Read the model definition and answer for the solid it produces. Units are mm, in the model's axes. Face numbers are marked on the shaded views. Coordinates: 2 decimals unless noted, no trailing zeros. Loops run counter-clockwise (first coordinate to the right, second up) from the corner with the lowest first, then second, coordinate; pieces in that order, holes last. Notation, with made-up numbers: M 43.25,-6 L 86.25,-6 A18 cw 86.25,-2 Z; hole C 44,58 d9. An arc over 180 degrees is marked long. Use one line per item in the form item = value. Start each with the question number.
1. The part is cut by section B-B (y = 32.5). Give the vertices of the cut face in (x, z).
2. Find the intervals of material crossed by probe 1 along Y at (x, z) = (-2.05, 0); probe 2 along Y at (x, z) = (-2.25, 1.25); probe 3 along X at (y, z) = (32, -1.75), in increasing order. Write a range as [from, to].
3. The part is cut by section D-D (y = 23). Give the vertices of the cut face in (x, z), plus the area to 3 significant figures.
4. For a pull along X with two mould halves and no side action, classify the marked faces 1 and 2 as released by +X, released by -X, zero draft, split by the parting line, or undercut.
5. The part is cut by section A-A (y = -2.5). Give the number of separate pieces and of enclosed holes in the cut face, plus the area to 3 significant figures.
6. Flat-ended cylindrical pins translate along their axes: pin 1 (2.5 mm diameter, centred on y = 32.5, z = 0, fed in from -X); pin 2 (3 mm diameter, centred on y = 18.5, z = -2.5, fed in from -X); pin 3 (2.5 mm diameter, centred on x = -0.5, z = 0.5, fed in from +Y); pin 4 (0.6 mm diameter, centred on y = -3, z = -2.5, fed in from -X). Find the tip coordinate at first contact, or state that the pin passes through.
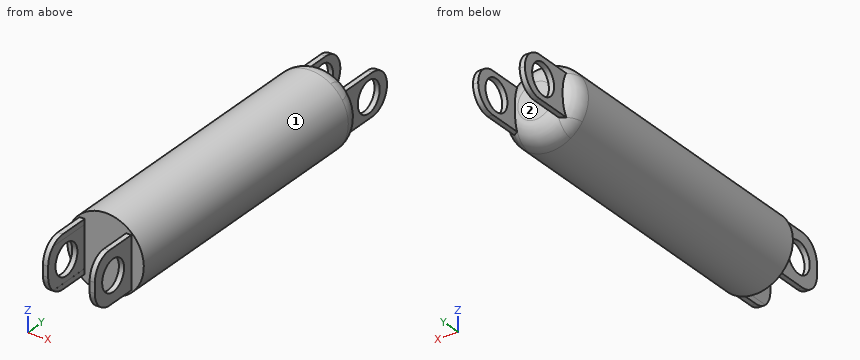
from build123d import *

# Parameters (mm, degrees)
SKETCH1_R           = 3.7
BOSS_EXTRUDE1_DEPTH = 30
SKETCH2_W           = 5
SKETCH2_H           = 4
SKETCH2_W_2         = 4
SKETCH2_H_2         = 3
BOSS_EXTRUDE2_DEPTH = 5
SKETCH3_W           = 4
SKETCH3_H           = 4.53219821
CUT_EXTRUDE1_DEPTH  = 5
SKETCH4_R           = 1.5
CUT_EXTRUDE2_DEPTH  = 15
FILLET1_R           = 2
FILLET2_R           = 2
SKETCH5_W           = 5
SKETCH5_H           = 5
SKETCH5_W_2         = 4
SKETCH5_H_2         = 4
BOSS_EXTRUDE3_DEPTH = 5
SKETCH6_W           = 3.994620944
SKETCH6_H           = 5.818695304
CUT_EXTRUDE3_DEPTH  = 5
SKETCH7_R           = 1.5
CUT_EXTRUDE4_DEPTH  = 5
FILLET3_R           = 2


# Some blends are built 0.0001 mm under size
with BuildPart() as part:
    # Sketch1 → Boss-Extrude1 (new body)
    with BuildSketch(Plane(origin=(0, 0, 0), x_dir=(1, 0, 0), z_dir=(0, 1, 0))):
        with Locations(Location((0, 0, 0), (0, 0, 270))):
            Circle(SKETCH1_R)
    extrude(amount=BOSS_EXTRUDE1_DEPTH)

    # Sketch2 → Boss-Extrude2 (add)
    with BuildSketch(Plane(origin=(0, 30, 0), x_dir=(1, 0, 0), z_dir=(0, 1, 0))):
        Rectangle(SKETCH2_W, SKETCH2_H)
        Rectangle(SKETCH2_W_2, SKETCH2_H_2, mode=Mode.SUBTRACT)
    extrude(amount=BOSS_EXTRUDE2_DEPTH)

    # Sketch3 → Cut-Extrude1 (cut)
    with BuildSketch(Plane(origin=(0, 35, 0), x_dir=(1, 0, 0), z_dir=(0, 1, 0))):
        Rectangle(SKETCH3_W, SKETCH3_H)
    extrude(amount=-CUT_EXTRUDE1_DEPTH, mode=Mode.SUBTRACT)

    # Sketch4 → Cut-Extrude2 (cut)
    with BuildSketch(Plane.ZY.offset(2.5)):
        with Locations((0, 32.5)):
            Circle(SKETCH4_R)
    extrude(amount=-CUT_EXTRUDE2_DEPTH, mode=Mode.SUBTRACT)

    # Fillet1
    fillet1_edges = [part.edges().sort_by_distance(p)[0] for p in [
        (-2.25, 35, 2),
        (-2.25, 35, -2),
        (2.25, 35, -2),
        (2.25, 35, 2),
    ]]
    fillet(fillet1_edges, radius=FILLET1_R - 0.0001)  # a hair under: the kernel refuses the full size

    # Fillet2
    # the kernel refuses this fillet: 2 mm, written as the material it takes off along each edge
    with BuildSketch(Plane(origin=(0, 30, 0), x_dir=(0, 0, 1), z_dir=(-1, 0, 0))) as fillet2_piece_1_section:
        with BuildLine():
            CenterArc((3.7 - FILLET2_R, -FILLET2_R), FILLET2_R, 0, 90)
            Line((3.7, -FILLET2_R), (3.7, 0))
            Line((3.7, 0), (3.7 - FILLET2_R, 0))
        make_face()
    fillet2_piece_1 = revolve(axis=Axis((0, 30, 0), (0, 1, 0)), mode=Mode.PRIVATE)
    fillet2_piece_1 = split(fillet2_piece_1, bisect_by=Plane(origin=(2, 29.996904363, 0.950092039), z_dir=(-1, 0, 0)), keep=Keep.TOP, mode=Mode.PRIVATE)
    fillet2_piece_1 = split(fillet2_piece_1, bisect_by=Plane(origin=(-2, 29.996904363, 0.950092039), z_dir=(1, 0, 0)), keep=Keep.TOP, mode=Mode.PRIVATE)
    add(fillet2_piece_1, mode=Mode.SUBTRACT)
    with BuildSketch(Plane(origin=(0, 30, 0), x_dir=(0, 0, 1), z_dir=(-1, 0, 0))) as fillet2_piece_2_section:
        with BuildLine():
            CenterArc((3.7 - FILLET2_R, -FILLET2_R), FILLET2_R, 0, 90)
            Line((3.7, -FILLET2_R), (3.7, 0))
            Line((3.7, 0), (3.7 - FILLET2_R, 0))
        make_face()
    fillet2_piece_2 = revolve(axis=Axis((0, 30, 0), (0, 1, 0)), mode=Mode.PRIVATE)
    fillet2_piece_2 = split(fillet2_piece_2, bisect_by=Plane(origin=(2.24397726, 29.466228533, 2), z_dir=(0, 0, 1)), keep=Keep.TOP, mode=Mode.PRIVATE)
    add(fillet2_piece_2, mode=Mode.SUBTRACT)
    with BuildSketch(Plane(origin=(0, 30, 0), x_dir=(0, 0, 1), z_dir=(-1, 0, 0))) as fillet2_piece_3_section:
        with BuildLine():
            CenterArc((3.7 - FILLET2_R, -FILLET2_R), FILLET2_R, 0, 90)
            Line((3.7, -FILLET2_R), (3.7, 0))
            Line((3.7, 0), (3.7 - FILLET2_R, 0))
        make_face()
    fillet2_piece_3 = revolve(axis=Axis((0, 30, 0), (0, 1, 0)), mode=Mode.PRIVATE)
    fillet2_piece_3 = split(fillet2_piece_3, bisect_by=Plane(origin=(2.5, 29.502863649, 1.19e-07), z_dir=(1, 0, 0)), keep=Keep.TOP, mode=Mode.PRIVATE)
    add(fillet2_piece_3, mode=Mode.SUBTRACT)
    with BuildSketch(Plane(origin=(0, 30, 0), x_dir=(0, 0, 1), z_dir=(-1, 0, 0))) as fillet2_piece_4_section:
        with BuildLine():
            CenterArc((3.7 - FILLET2_R, -FILLET2_R), FILLET2_R, 0, 90)
            Line((3.7, -FILLET2_R), (3.7, 0))
            Line((3.7, 0), (3.7 - FILLET2_R, 0))
        make_face()
    fillet2_piece_4 = revolve(axis=Axis((0, 30, 0), (0, 1, 0)), mode=Mode.PRIVATE)
    fillet2_piece_4 = split(fillet2_piece_4, bisect_by=Plane(origin=(2.243977257, 29.466228303, -2), z_dir=(0, 0, -1)), keep=Keep.TOP, mode=Mode.PRIVATE)
    add(fillet2_piece_4, mode=Mode.SUBTRACT)
    with BuildSketch(Plane(origin=(0, 30, 0), x_dir=(0, 0, 1), z_dir=(-1, 0, 0))) as fillet2_piece_5_section:
        with BuildLine():
            CenterArc((3.7 - FILLET2_R, -FILLET2_R), FILLET2_R, 0, 90)
            Line((3.7, -FILLET2_R), (3.7, 0))
            Line((3.7, 0), (3.7 - FILLET2_R, 0))
        make_face()
    fillet2_piece_5 = revolve(axis=Axis((0, 30, 0), (0, 1, 0)), mode=Mode.PRIVATE)
    fillet2_piece_5 = split(fillet2_piece_5, bisect_by=Plane(origin=(-2.5, 29.50286365, -1.18e-07), z_dir=(-1, 0, 0)), keep=Keep.TOP, mode=Mode.PRIVATE)
    add(fillet2_piece_5, mode=Mode.SUBTRACT)

    # Sketch5 → Boss-Extrude3 (add)
    with BuildSketch(Plane.XZ):
        Rectangle(SKETCH5_W, SKETCH5_H)
        Rectangle(SKETCH5_W_2, SKETCH5_H_2, mode=Mode.SUBTRACT)
    extrude(amount=BOSS_EXTRUDE3_DEPTH)

    # Sketch6 → Cut-Extrude3 (cut)
    with BuildSketch(Plane.XZ.offset(5)):
        Rectangle(SKETCH6_W, SKETCH6_H)
    extrude(amount=-CUT_EXTRUDE3_DEPTH, mode=Mode.SUBTRACT)

    # Sketch7 → Cut-Extrude4 (cut)
    with BuildSketch(Plane(origin=(2.5, 0, 0), x_dir=(0, 0, -1), z_dir=(1, 0, 0))):
        with Locations((0, -2.5)):
            Circle(SKETCH7_R)
    extrude(amount=-CUT_EXTRUDE4_DEPTH, mode=Mode.SUBTRACT)

    # Fillet3
    fillet3_edges = [part.edges().sort_by_distance(p)[0] for p in [
        (-2.248655236, -5, -2.5),
        (-2.248655236, -5, 2.5),
        (2.248655236, -5, 2.5),
        (2.248655236, -5, -2.5),
    ]]
    fillet(fillet3_edges, radius=FILLET3_R)


solid = part.part
Computed values:
q1.outline = M -2.5,-2 L -2,-2 L -2,-1.5 L -2.5,-1.5 Z; M -2.5,1.5 L -2,1.5 L -2,2 L -2.5,2 Z; M 2,-2 L 2.5,-2 L 2.5,-1.5 L 2,-1.5 Z; M 2,1.5 L 2.5,1.5 L 2.5,2 L 2,2 Z
q2.probe_1 = [-5, -4], [-1, 31], [34, 35]
q2.probe_2 = [-4.85, -3.33], [-1.67, 31.67], [33.33, 34.56]
q2.probe_3 = [-2.5, -2], [2, 2.5]
q3.outline = C 0,0 d7.4
q3.area = 43.0 mm²
q4.face_1 = split by the parting line
q4.face_2 = undercut
q5.separate_pieces = 4
q5.enclosed_holes = 0
q5.area = 2.01 mm²
q6.pin_1 = through
q6.pin_2 = -3.56
q6.pin_3 = 30
q6.pin_4 = -2.5
